Job drawing, mm, ordinate dimensions from the low corner. One solid piece. A direction names the side the tool comes from. Give positions to 0.01 mm unless a question says otherwise; leave off trailing zeros. Order: outer loops, then holes, each group sorted by start corner. A loop starts at its lowest first (then second) coordinate and runs counter-clockwise, first axis right, second up.
1. Drop flat-ended pins along their axis: pin 1 Ø6 at (y, z) = (5.5, 7) entering from +X; pin 2 Ø3 at (x, z) = (7.25, 2) entering from -Y; pin 3 Ø1.8 at (x, y) = (5, 33.5) entering from +Z; pin 4 Ø7 at (x, y) = (7, 20.5) entering from -Z. Give the stop position or say it passes through.
2. Slice it at C-C on x = 5.25. List the corners of the cut face in (y, z).
3. Which spindle directions (+Z, -Z, +X, -X, +Y, -Y) get a long thin tool onto all of the face, cutting with end or side? Do the marked faces 1, 2 and 3. Say none if no direction does.
4. Slice it at D-D on x = 7.25. List the corners of the cut face in (y, z), and give its area (3 significant figures).
5. Probe line 1 (Y direction, x = 7.25, z = 12.4); line 2 (X direction, y = 1.2, z = 2); line 3 (X direction, y = 31, z = 14.25). List the from-to ranges inside material, lowest first.
6. Slice it at B-B on y = 4. List the corners of the cut face in (x, z).
7. Slice it at A-A on z = 2. List the corners of the cut face in (x, y), and give its area (3 significant figures).
8. Mould opens along X. For the marked faces 4, 5 and 6 say: +X half, -X half, draft (parallel to the pull), parting line (faces both ways), or undercut.
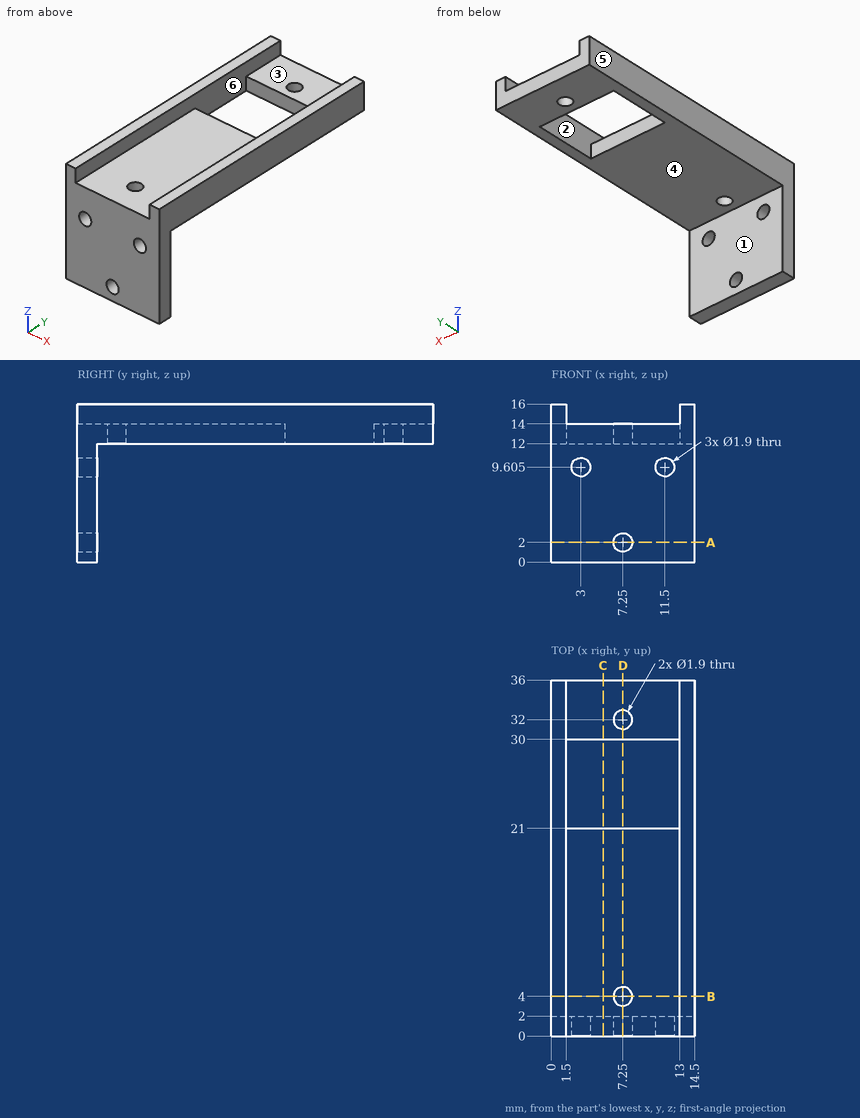
Data:
1. pin 1: passes through
1. pin 2: stops at y = 0
1. pin 3: stops at z = 14
1. pin 4: stops at z = 12
2. outline: (0, 0) - (2, 0) - (2, 12) - (21, 12) - (21, 14) - (0, 14) - close; (30, 12) - (36, 12) - (36, 14) - (30, 14) - close
3. face 1: -Z, +X, -X, +Y
3. face 2: +Z
3. face 3: +Z, +Y, -Y
4. outline: (0, 0) - (2, 0) - (2, 1.05) - (0, 1.05) - close; (0, 2.95) - (2, 2.95) - (2, 12) - (3.05, 12) - (3.05, 14) - (0, 14) - close; (4.95, 12) - (21, 12) - (21, 14) - (4.95, 14) - close; (30, 12) - (31.05, 12) - (31.05, 14) - (30, 14) - close; (32.95, 12) - (36, 12) - (36, 14) - (32.95, 14) - close
4. area: 66.6 mm2
5. line 1: y = 0 to 3.05, 4.95 to 21, 30 to 31.05, 32.95 to 36
5. line 2: x = 0 to 6.3, 8.2 to 14.5
5. line 3: x = 0 to 1.5, 13 to 14.5
6. outline: (0, 12) - (6.3, 12) - (6.3, 14) - (1.5, 14) - (1.5, 16) - (0, 16) - close; (8.2, 12) - (14.5, 12) - (14.5, 16) - (13, 16) - (13, 14) - (8.2, 14) - close
7. outline: (0, 0) - (6.3, 0) - (6.3, 2) - (0, 2) - close; (8.2, 0) - (14.5, 0) - (14.5, 2) - (8.2, 2) - close
7. area: 25.2 mm2
8. face 4: draft
8. face 5: -X half
8. face 6: undercut
